Verification items for this drawing (mm, ordinates from the low corner). Round coordinates to 2 decimals unless told otherwise and drop trailing zeros. Order: outer loops, then holes, each group sorted by start corner. A loop starts at its lowest first (then second) coordinate and runs counter-clockwise, first axis right, second up.
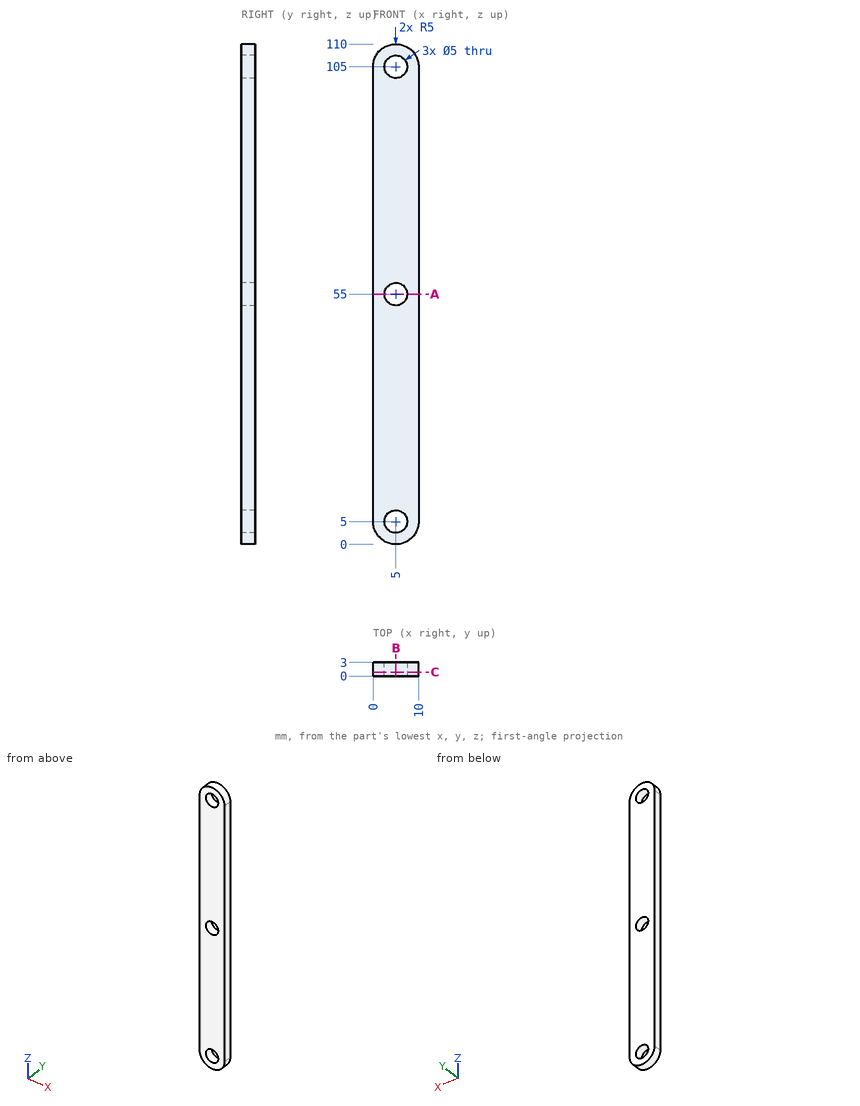
Item 1: Sectioned sample at B-B (x = 5). Record the cut outline in (y, z).
Answer:
outline: (0, 0) - (3, 0) - (3, 2.5) - (0, 2.5) - close; (0, 7.5) - (3, 7.5) - (3, 52.5) - (0, 52.5) - close; (0, 57.5) - (3, 57.5) - (3, 102.5) - (0, 102.5) - close; (0, 107.5) - (3, 107.5) - (3, 110) - (0, 110) - close
Item 2: Sectioned sample at C-C (y = 0.85). Record the cut outline in (x, z), and give its area (3 significant figures).
Answer:
outline: (0, 5) arc R5 ccw to (10, 5) - (10, 105) arc R5 ccw to (0, 105) - close; hole circle Ø5 at (5, 5); hole circle Ø5 at (5, 55); hole circle Ø5 at (5, 105)
area: 1,020 mm2
Item 3: Go/stop test with flat-tipped pins: P1, Ø1, axis at x = 6, y = 0.5, coming from the -Z side; P2, Ø1, axis at x = 8.5, y = 1.5, coming from the +Z side. Record where each tip stops, or that it passes through.
Answer:
P1: stops at z = 0.03
P2: stops at z = 109
Item 4: Sectioned sample at A-A (z = 55). Record the cut outline in (x, y).
Answer:
outline: (0, 0) - (2.5, 0) - (2.5, 3) - (0, 3) - close; (7.5, 0) - (10, 0) - (10, 3) - (7.5, 3) - close
Item 5: Scan lines: line 1 along Z through (x, y) = (5, 1.1); line 2 along Z through (x, y) = (5.5, 1.95); line 3 along X through (y, z) = (0.8, 105.5). Record each from-to range of solid material in increasing order.
Answer:
line 1: z = 0 to 2.5, 7.5 to 52.5, 57.5 to 102.5, 107.5 to 110
line 2: z = 0.03 to 2.55, 7.45 to 52.55, 57.45 to 102.55, 107.45 to 109.97
line 3: x = 0.03 to 2.55, 7.45 to 9.97
